Autodesk Inventor part; units mm, degrees
ref_plane "YZ Plane" through (0, 0, 0) normal (1, 0, 0) x (0, 1, 0)
ref_plane "XZ Plane" through (0, 0, 0) normal (0, 1, 0) x (-1, 0, 0)
ref_plane "XY Plane" through (0, 0, 0) normal (0, 0, 1) x (1, 0, 0)
sketch "Sketch1" plane through (0, 0, 0) normal (0, 0, 1) x (1, 0, 0)
  circle A0 centre (0, 0) radius 40
  circle A1 centre (0, 0) radius 10
  dimension "d0" = 80
  dimension "d1" = 20
extrude "Extrusion1" add sketch "Sketch1" along normal blind 24
fillet "Fillet1" radius 11.938 2 edges at (-40, 0, 24) (-40, 0, 0)
sketch "Sketch2" plane through (0, 0, 24) normal (0, 0, 1) x (1, 0, 0)
  circle A0 centre (0, 0) radius 11
  circle A1 centre (0, 0) radius 10
  dimension "d5" = 22
extrude "Extrusion2" cut sketch "Sketch2" against normal blind 7
sketch "Sketch3" plane through (0, 0, 0) normal (0, 0, -1) x (-1, 0, 0)
  circle A0 centre (0, 0) radius 11
  circle A1 centre (0, 0) radius 10
  dimension "d8" = 22
  dimension "d9" = 20
extrude "Extrusion3" cut sketch "Sketch3" against normal blind 7
properties part number "wheel_80mm"
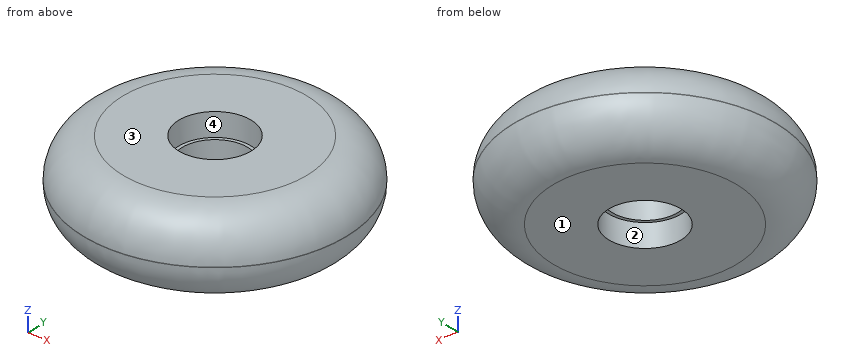
Geometry: final body of the model. Coordinates: model frame, mm. Face numbers are marked on the shaded views. A direction names the side the tool comes from. Round coordinates to 2 decimals unless told otherwise and drop trailing zeros. Loops run counter-clockwise (first coordinate to the right, second up) from the corner with the lowest first, then second, coordinate; pieces in that order, holes last. Notation, with made-up numbers: (59, 35.25) -> (111, 35.25) arc R17 ccw to (111, 68.25) -> close; hole circle Ø9 at (51.5, 17.5). An arc over 180 degrees is marked (long way). Write each question's results on one line, items separated by ' | '.
Item 1: Cut plane A-A on y = 0. Return the cut outline in (x, z), and give its area (3 significant figures).
Answers below:
outline: (-40, 11.94) arc R11.94 ccw to (-28.06, 0) -> (-11, 0) -> (-11, 7) -> (-10, 7) -> (-10, 17) -> (-11, 17) -> (-11, 24) -> (-28.06, 24) arc R11.94 ccw to (-40, 12.06) -> close; (10, 7) -> (11, 7) -> (11, 0) -> (28.06, 0) arc R11.94 ccw to (40, 11.94) -> (40, 12.06) arc R11.94 ccw to (28.06, 24) -> (11, 24) -> (11, 17) -> (10, 17) -> close | area: 1,290 mm²
Item 2: Pull-direction query (Y, two-part tool) for the marked faces 1 and 2; classes: pulls with the +Y half, pulls with the -Y half, needs draft (parallel to the pull), parting line crosses it, or undercut.
Answers below:
face 1: needs draft | face 2: undercut
Item 3: Pin query (flat end, axial travel): pin 1 Ø3 at (x, z) = (1.5, 15.5) entering from +Y; pin 2 Ø2 at (x, y) = (14, -27.5) entering from +Z; pin 3 Ø12 at (x, y) = (15, 27.5) entering from +Z; pin 4 Ø11 at (x, y) = (3.5, -3) entering from +Z. Return the tip coordinate at first contact, or that it passes through.
Answers below:
pin 1: stops at y = 39.82 | pin 2: stops at z = 23.86 | pin 3: stops at z = 24 | pin 4: stops at z = 17
Item 4: Cut plane D-D on z = 8. Return the cut outline in (x, y).
Answers below:
outline: circle Ø78.66 at (0, 0); hole circle Ø20 at (0, 0)
Item 5: Set-up query: the marked faces 3 and 4. Return all of +Z, -Z, +X, -X, +Y, -Y with unobstructed straight access to the full face (end or side cutting, diameter ignored); none if empty.
Answers below:
face 3: +Z, +X, -X, +Y, -Y | face 4: +Z
Item 6: Line query: probe 1 along Y at (x, z) = (0, 11.75); probe 2 along Y at (x, z) = (0, 20); probe 3 along X at (y, z) = (2, 14.75). Output: solid intervals per line, ascending. Write a range as [from, to].
Answers below:
probe 1: y = [-40, -10], [10, 40] | probe 2: y = [-36.98, -11], [11, 36.98] | probe 3: x = [-39.64, -9.8], [9.8, 39.64]
Item 7: Cut plane C-C on z = 13. Return the cut outline in (x, y), and give its area (3 significant figures).
Answers below:
outline: circle Ø79.93 at (0, 0); hole circle Ø20 at (0, 0) | area: 4,700 mm²
